Could you check a few things on this model? Use its own coordinates, in mm. Coordinates: 2 decimals unless noted, no trailing zeros. Order: outer loops, then holes, each group sorted by start corner. A loop starts at its lowest first (then second) coordinate and runs counter-clockwise, first axis right, second up. Notation, with made-up numbers: (66.5, 26.25) - (96.5, 26.25) arc R10 ccw to (96.5, 35.25) - close; hole circle Ø6 at (14, 40.25). An arc over 180 degrees is marked (long way). One line per item, written item: value.
from build123d import *

# Parameters (mm, degrees)
F2_R     = 3.733432
F2_R_2   = 3.5
F2_R_3   = 3.61173
F3_DEPTH = 25
F4_R     = 10


with BuildPart() as f1:
    # F0 (on Front) → F1 (revolve)
    with BuildSketch(Plane.XZ):
        with BuildLine():
            Line((0, 13.896797), (0, 19.229659))
            Line((0, 19.229659), (-9, 19.229659))
            Line((-9, 19.229659), (-9, 16.896797))
            ThreePointArc((-9, 16.896797), (-4.743416, 14.666548), (0, 13.896797))
        make_face()
        with BuildLine():
            Line((-9, 19.229659), (0, 19.229659))
            Line((0, 19.229659), (0, 43.896797))
            ThreePointArc((0, 43.896797), (-14.230249, 33.640214), (-9, 16.896797))
            Line((-9, 16.896797), (-9, 19.229659))
        make_face()
        with BuildLine():
            Line((0, -5.770341), (0, 13.896797))
            ThreePointArc((0, 13.896797), (-4.743416, 14.666548), (-9, 16.896797))
            Line((-9, 16.896797), (-9, -5.770341))
            Line((-9, -5.770341), (0, -5.770341))
        make_face()
        Polygon((0, -13.677974), (0, -5.770341), (-9, -5.770341), (-30, -5.770341), (-30, -15.770341), (0, -15.770341), align=None)
    revolve(axis=Axis((0, 0, 17.993038), (0, 0, -1)))

    # F2 (on face) → F3 (cut)
    with BuildSketch(Plane(origin=(0, 0, -15.770341), x_dir=(1, 0, 0), z_dir=(0, 0, -1))):
        with Locations((-17, 17)):
            Circle(F2_R)
        with Locations((17, 17)):
            Circle(F2_R_2)
        with Locations((-17, -17)):
            Circle(F2_R_3)
        with Locations((17, -17)):
            Circle(F2_R_2)
    extrude(amount=-F3_DEPTH, mode=Mode.SUBTRACT)

    # F4
    f4_edges = [f1.edges().sort_by_distance(p)[0] for p in [
        (9, 0, -5.770341),
    ]]
    fillet(f4_edges, radius=F4_R)


solid = f1.part
Item 1: Thinking about a two-plate mould opening in Z: for faces 1 (the face through (0, 0, -15.77)), 2 (the face through (0, -20, -5.77)), 3 (the face through (-13.44, -18.12, -10.84)), 4 (the face through (1.172, 8.923, 10.475)), which applies, pulls with the +Z half, pulls with the -Z half, needs draft (parallel to the pull), parting line crosses it, or undercut?
Conclusion:
face 1: pulls with the -Z half
face 2: pulls with the +Z half
face 3: needs draft
face 4: undercut
Item 2: If I drill on probe 1 along Y at (x, z) = (-17, -11); probe 2 along Y at (x, z) = (17, -13); probe 3 along X at (y, z) = (17, -13.25), over which ranges is the centre line in solid material (lowest first)?
Conclusion:
probe 1: -24.72 to -20.73, -13.27 to 13.39, 20.61 to 24.72
probe 2: -24.72 to -20.5, -13.5 to 13.5, 20.5 to 24.72
probe 3: -24.72 to -20.61, -13.39 to 13.5, 20.5 to 24.72
Item 3: I'm going to push flat-ended pins straight in: pin 1 Ø1.5 at (x, y) = (7.5, -9) entering from +Z; pin 2 Ø6 at (y, z) = (17.5, -5.5) entering from -X; pin 3 Ø4 at (x, y) = (15.5, -18) entering from +Z; pin 4 Ø6.5 at (x, y) = (17, -17) entering from -Z. Where does each tip first touch, or does it pass through?
Conclusion:
pin 1: z = 39.13
pin 2: x = -26.26
pin 3: z = -5.77
pin 4: through
Item 4: I want a section at C-C on y = 24. Please give me the cut outline in (x, z).
Conclusion:
outline: (-18, -15.77) - (18, -15.77) - (18, -5.77) - (-18, -5.77) - close
Item 5: I want a section at A-A on x = 17. Give the number of separate pieces and of enclosed holes in the cut face, then the cut area to 3 significant figures.
Conclusion:
separate pieces: 3
enclosed holes: 0
area: 356 mm²
